The model under review builds one solid part; all positions refer to its coordinate system, in mm. A direction names the side the tool comes from. Give positions to 0.01 mm unless a question says otherwise; leave off trailing zeros. Loops run counter-clockwise (first coordinate to the right, second up) from the corner with the lowest first, then second, coordinate; pieces in that order, holes last. Notation, with made-up numbers: M 30,65.25 L 84,65.25 A31 cw 84,104.25 Z; hole C -35.5,76.25 d9. An arc over 180 degrees is marked long. Return JSON: item names as keys, results as strings. Group by question number.
```python
from build123d import *

# Parameters (mm, degrees)
SKETCH_1_W          = 50
SKETCH_1_H          = 68
SKETCH_1_R          = 0.5
SKETCH_1_W_2        = 43
SKETCH_1_H_2        = 61
EXTRUDE_1_DEPTH     = 3
FILLET_1_R          = 2
SKETCH_1_5_R        = 0.5
CUT_EXTRUDE_1_DEPTH = 2
FILLET_2_R          = 0.6
CHAMFER_1_SIZE      = 1


with BuildPart() as part:
    # Sketch 1 → Extrude 1 (new body)
    # profile 1 of 5: a face of its own
    with BuildSketch(Plane.XY):
        Rectangle(SKETCH_1_W, SKETCH_1_H)
        with Locations((-23, -32)):
            Circle(SKETCH_1_R, mode=Mode.SUBTRACT)
        with Locations((23, -32)):
            Circle(SKETCH_1_R, mode=Mode.SUBTRACT)
        with Locations((23, 32)):
            Circle(SKETCH_1_R, mode=Mode.SUBTRACT)
        with Locations((-23, 32)):
            Circle(SKETCH_1_R, mode=Mode.SUBTRACT)
        Rectangle(SKETCH_1_W_2, SKETCH_1_H_2, mode=Mode.SUBTRACT)
    # profile 2 of 5: a face of its own
    with BuildSketch(Plane.XY):
        with Locations((23, -32)):
            Circle(SKETCH_1_R)
    # profile 3 of 5: a face of its own
    with BuildSketch(Plane.XY):
        with Locations((-23, -32)):
            Circle(SKETCH_1_R)
    # profile 4 of 5: a face of its own
    with BuildSketch(Plane.XY):
        with Locations((-23, 32)):
            Circle(SKETCH_1_R)
    # profile 5 of 5: a face of its own
    with BuildSketch(Plane.XY):
        with Locations((23, 32)):
            Circle(SKETCH_1_R)
    extrude(amount=EXTRUDE_1_DEPTH)

    # Fillet 1
    fillet_1_edges = [part.edges().sort_by_distance(p)[0] for p in [
        (-25, -34, 1.5),
        (-25, 34, 1.5),
        (25, 34, 1.5),
        (25, -34, 1.5),
    ]]
    fillet(fillet_1_edges, radius=FILLET_1_R)

    # Sketch 1_5 → Cut-Extrude 1 (cut)
    with BuildSketch(Plane.XY):
        with Locations((23, 32)):
            Circle(SKETCH_1_5_R)
        with Locations((-23, 32)):
            Circle(SKETCH_1_5_R)
        with Locations((-23, -32)):
            Circle(SKETCH_1_5_R)
        with Locations((23, -32)):
            Circle(SKETCH_1_5_R)
    extrude(amount=CUT_EXTRUDE_1_DEPTH, mode=Mode.SUBTRACT)

    # Fillet 2
    fillet_2_edges = [part.edges().sort_by_distance(p)[0] for p in [
        (0, -34, 3),
        (-25, 0, 3),
        (25, 0, 3),
        (0, 34, 3),
        (-24.414213562, 33.414213562, 3),
        (24.414213562, 33.414213562, 3),
        (24.414213562, -33.414213562, 3),
        (-24.414213562, -33.414213562, 3),
    ]]
    fillet(fillet_2_edges, radius=FILLET_2_R)

    # Chamfer 1
    chamfer_1_edges = [part.edges().sort_by_distance(p)[0] for p in [
        (0, -30.5, 3),
        (-21.5, 0, 3),
        (0, 30.5, 3),
        (21.5, 0, 3),
    ]]
    chamfer(chamfer_1_edges, length=CHAMFER_1_SIZE)


solid = part.part
```
(1) For pin 1 (0.5 mm diameter, centred on x = -23, y = 32, fed in from -Z), flat-tipped, find the tip position at first contact; note if it passes through.
(2) For probe 1 along Y at (x, z) = (23, 1.6); probe 2 along X at (y, z) = (32, 0.8); probe 3 along X at (y, z) = (-6, 0.5), list the stretches that pass through material, from the lowest coordinate up.
(3) Mouldability with a two-part tool opening along X and no side actions: class faces 1 (the cylindrical face through (-24.43, -33.4, 1.22)), 2 (the flat face through (0, 30.5, 1)), 3 (the flat face through (-22, 3, 0)) as released by +X, released by -X, zero draft, split by the parting line, or undercut.
(4) For faces 4 (the flat face through (0, -30.5, 1)), 5 (the cylindrical face through (-24.43, 33.4, 1.22)), list the 3-axis set-ups (+Z, -Z, +X, -X, +Y, -Y) from which the entire face can be reached by the end or side of a thin tool; tool diameter is ignored.
(5) Add section A-A (x = -17.5). Write out the cut boundary in (y, z).
(6) Add section B-B (z = 0.6). Write out the cut boundary in (x, y).
(7) Add section C-C (y = -24). Write out the cut boundary in (x, z).
Verdict:
{
 "1": {"pin 1": "stops at z = 2"},
 "2": {"probe 1": "y = -34 to -32.5, -31.5 to 31.5, 32.5 to 34", "probe 2": "x = -25 to -23.5, -22.5 to 22.5, 23.5 to 25", "probe 3": "x = -25 to -21.5, 21.5 to 25"},
 "3": {"face 1": "released by -X", "face 2": "undercut", "face 3": "zero draft"},
 "4": {"face 4": "+Z, -Z", "face 5": "+Z, -Z, -X, +Y"},
 "5": {"outline": "M -34,0 L -30.5,0 L -30.5,2 L -31.5,3 L -33.4,3 A0.6 ccw -34,2.4 Z; M 30.5,0 L 34,0 L 34,2.4 A0.6 ccw 33.4,3 L 31.5,3 L 30.5,2 Z"},
 "6": {"outline": "M -25,-32 A2 ccw -23,-34 L 23,-34 A2 ccw 25,-32 L 25,32 A2 ccw 23,34 L -23,34 A2 ccw -25,32 Z; hole C -23,-32 d1; hole C -23,32 d1; hole M -21.5,-30.5 L 21.5,-30.5 L 21.5,30.5 L -21.5,30.5 Z; hole C 23,-32 d1; hole C 23,32 d1"},
 "7": {"outline": "M -25,0 L -21.5,0 L -21.5,2 L -22.5,3 L -24.4,3 A0.6 ccw -25,2.4 Z; M 21.5,0 L 25,0 L 25,2.4 A0.6 ccw 24.4,3 L 22.5,3 L 21.5,2 Z"}
}
